from build123d import *

# Parameters (mm, degrees)
F0_W     = 6.35
F0_H     = 6.35
F0_H_2   = 38.1
F0_W_2   = 127
F1_DEPTH = 12.7
F2_DEPTH = 3.175
F3_DEPTH = 3.175
F4_R     = 3.175


with BuildPart() as f1:
    # F0 (on Top) → F1 (new body)
    with BuildSketch(Plane.XY):
        with Locations((71.6993232399, -31.2760059339)):
            Rectangle(F0_W, F0_H)
        with Locations((-61.6506767601, -9.0510059339)):
            Rectangle(F0_W, F0_H_2)
        with Locations((-61.6506767601, 13.1739940661)):
            Rectangle(F0_W, F0_H)
        with Locations((5.0243232399, 13.1739940661)):
            Rectangle(F0_W_2, F0_H)
        with Locations((71.6993232399, -9.0510059339)):
            Rectangle(F0_W, F0_H_2)
        with Locations((71.6993232399, 13.1739940661)):
            Rectangle(F0_W, F0_H)
        with Locations((5.0243232399, -31.2760059339)):
            Rectangle(F0_W_2, F0_H)
        with Locations((-61.6506767601, -31.2760059339)):
            Rectangle(F0_W, F0_H)
    extrude(amount=F1_DEPTH)

    # F2 (add): a face of the model
    f2_faces = [f1.faces().sort_by_distance(p)[0] for p in [
        (-63.3391798714, -9.0510059339, 0),
    ]]
    extrude(f2_faces, amount=F2_DEPTH)

    # F0 (on Top) → F3 (join)
    with BuildSketch(Plane.XY):
        Polygon((68.5243232399, 9.9989940661), (-58.4756767601, 9.9989940661), (68.5243232399, -28.1010059339), align=None)
        Polygon((68.5243232399, -28.1010059339), (-58.4756767601, 9.9989940661), (-58.4756767601, -28.1010059339), align=None)
    extrude(amount=-F3_DEPTH)

    # F4
    f4_edges = [f1.edges().sort_by_distance(p)[0] for p in [
        (-64.825677, -34.451006, 4.7625),
        (-64.825677, 16.348994, 4.7625),
        (74.874323, -34.451006, 4.7625),
        (74.874323, 16.348994, 4.7625),
    ]]
    fillet(f4_edges, radius=F4_R)


solid = f1.part
Source: CAD feature listing. Evaluate the final solid. Frame: model axes, mm. A direction names the side the tool comes from. Coordinates: 2 decimals unless noted, no trailing zeros. Write each loop counter-clockwise with the first axis right and the second up, starting at its lowest first coordinate (ties: lowest second). Pieces come first, ordered by that corner, then holes. Notation, with made-up numbers: M 36,55 L 41,55 A12 ccw 41,69 Z; hole C -15.5,39.5 d6. An arc over 180 degrees is marked long. Use a Markdown table: item, result.
1) First-contact query: pin 1 Ø10 at (x, y) = (-16.5, -19.5) entering from +Z. Flat tip, straight axial feed; report the tip coordinate or a pass-through.
Conclusion:
| item | result |
|---|---|
| pin 1 | stops at z = 0 |
2) Ray query, L1, parallel to X at y = 4.5, z = 4.75; L2, parallel to Y at x = 13.5, z = 2.25; L3, parallel to Z at x = 48, y = -10 (3 decimals). Return the intervals inside material, ascending.
Conclusion:
| item | result |
|---|---|
| L1 | x = -64.83 to -58.48, 68.52 to 74.87 |
| L2 | y = -34.45 to -28.1, 10 to 16.35 |
| L3 | z = -3.175 to 0 |
3) Section C-C, the plane y = -26.5. Output: boundary loops of the cut face in (x, z) (3 decimals), then the cut area to 3 significant figures.
Conclusion:
| item | result |
|---|---|
| outline | M -64.826,-3.175 L 74.874,-3.175 L 74.874,12.7 L 68.524,12.7 L 68.524,0 L -58.476,0 L -58.476,12.7 L -64.826,12.7 Z |
| area | 605 mm^2 |
4) Mould query, pull axis Y, two halves, no side actions, for faces 1 (the flat face through (4, -9, 0)), 2 (the cylindrical face through (-63.92, -33.496, 4.874)), 3 (the flat face through (4, -9, -3.175)). Classes: pulls with the +Y half, pulls with the -Y half, needs draft (parallel to the pull), parting line crosses it, or undercut.
Conclusion:
| item | result |
|---|---|
| face 1 | undercut |
| face 2 | pulls with the -Y half |
| face 3 | needs draft |
5) Section B-B, the plane z = 4.5. Output: boundary loops of the cut face in (x, y) (3 decimals).
Conclusion:
| item | result |
|---|---|
| outline | M -64.826,-31.276 A3.175 ccw -61.651,-34.451 L 71.699,-34.451 A3.175 ccw 74.874,-31.276 L 74.874,13.174 A3.175 ccw 71.699,16.349 L -61.651,16.349 A3.175 ccw -64.826,13.174 Z; hole M -58.476,-28.101 L 68.524,-28.101 L 68.524,9.999 L -58.476,9.999 Z |
6) Section A-A, the plane x = -12. Output: boundary loops of the cut face in (y, z) (3 decimals).
Conclusion:
| item | result |
|---|---|
| outline | M -34.451,-3.175 L 16.349,-3.175 L 16.349,12.7 L 9.999,12.7 L 9.999,0 L -28.101,0 L -28.101,12.7 L -34.451,12.7 Z |
7) Reachability of faces 4 (the cylindrical face through (-63.92, 15.394, 4.651)), 5 (the flat face through (-58.476, -9, 6)) from +Z, -Z, +X, -X, +Y, -Y: full face, straight path, thin tool, end or side. Return the list, or none.
Conclusion:
| item | result |
|---|---|
| face 4 | +Z, -Z, -X, +Y |
| face 5 | +Z |
